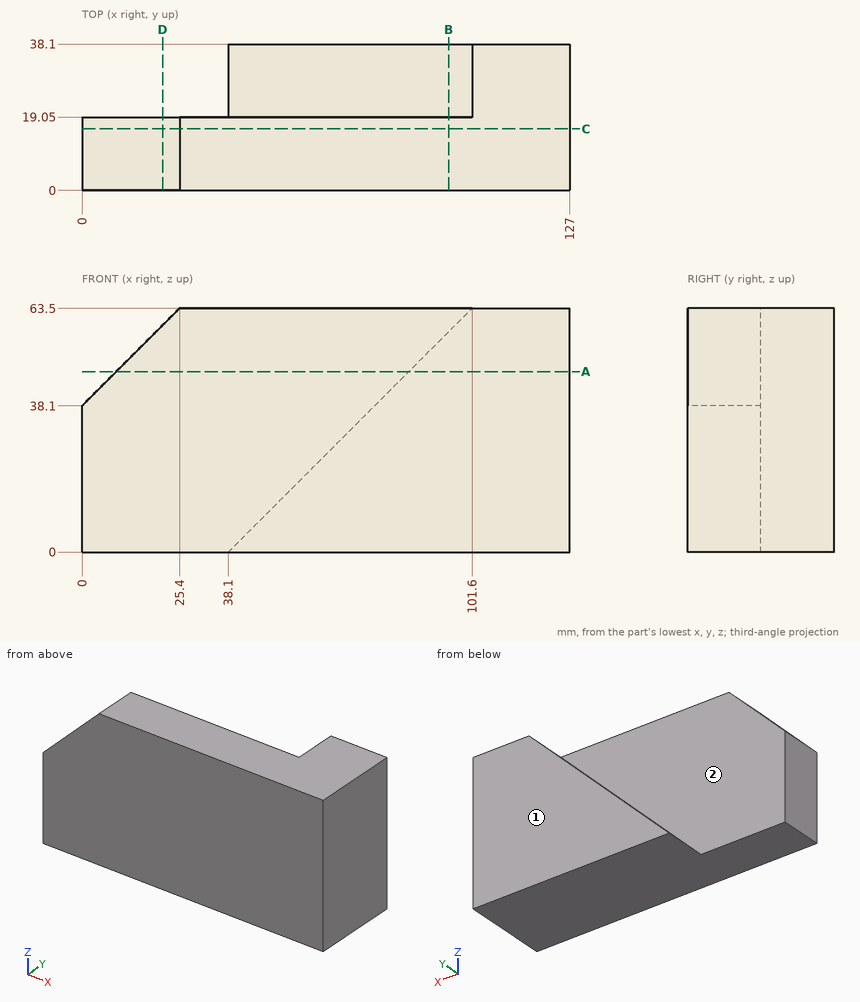
Study the drawing (mm; zero at the part's minimum x, y, z) and answer. A direction names the side the tool comes from. Round coordinates to 2 decimals unless told otherwise and drop trailing zeros. Loops run counter-clockwise (first coordinate to the right, second up) from the corner with the lowest first, then second, coordinate; pieces in that order, holes last. Notation, with made-up numbers: (40.25, -30) -> (57.25, -30) arc R13 ccw to (57.25, -13) -> close; hole circle Ø2 at (22, 77.5). An arc over 180 degrees is marked (long way). Use one line per item in the form item = value.
1. The part is cut by section B-B on x = 95.5. Determine the outline of the cut face in (y, z).
Answer key:
outline = (0, 0) -> (38.1, 0) -> (38.1, 57.4) -> (19.05, 57.4) -> (19.05, 63.5) -> (0, 63.5) -> close
2. A flat-ended cylindrical pin translates along its axis: pin 1 Ø19 at (x, z) = (40, 18) entering from +Y. Find the tip coordinate at first contact, or state that the pin passes through.
Answer key:
pin_1 = 19.05
3. A tool of negligible diameter and unlimited length cuts with its end or side. For the marked faces 1 and 2, from which of +Z, -Z, +X, -X, +Y, -Y can it reach the whole face along a straight path? Write none if from no direction.
Answer key:
face_1 = +Z, -Z, +X, -X, +Y
face_2 = +Z, -X, +Y
4. Find the intervals of material crossed by probe 1 along Y at (x, z) = (63, 39.5); probe 2 along X at (y, z) = (16, 39.5); probe 3 along X at (y, z) = (23.5, 41), in increasing order. Write a range as [from, to].
Answer key:
probe_1 = [0, 19.05]
probe_2 = [1.4, 127]
probe_3 = [79.1, 127]
5. The part is cut by section C-C on y = 16. Determine the outline of the cut face in (x, z), and give its area (3 significant figures).
Answer key:
outline = (0, 0) -> (127, 0) -> (127, 63.5) -> (25.4, 63.5) -> (0, 38.1) -> close
area = 7,740 mm²
6. The part is cut by section D-D on x = 21. Determine the outline of the cut face in (y, z), and give its area (3 significant figures).
Answer key:
outline = (0, 0) -> (19.05, 0) -> (19.05, 59.1) -> (0, 59.1) -> close
area = 1,130 mm²
7. The part is cut by section A-A on z = 47. Determine the outline of the cut face in (x, y).
Answer key:
outline = (8.9, 0) -> (127, 0) -> (127, 38.1) -> (85.1, 38.1) -> (85.1, 19.05) -> (8.9, 19.05) -> close
